from build123d import *

# Parameters (mm, degrees)
F0_W          = 10
F0_H          = 18
F1_DEPTH      = 25
F2_R          = 3.2
F3_DEPTH      = 50.401
F3_DEPTH_BACK = 35.001
F2_R_2        = 5.2
F4_DEPTH      = 5
F4_DEPTH_BACK = 35.001
F5_R          = 3.2
F6_DEPTH      = 5
F7_R          = 2
F8_SIZE       = 0.5


with BuildPart() as f1:
    # F0 (on Top) → F1 (new body)
    with BuildSketch(Plane.XY):
        Polygon((-15.2, 15.2), (15.2, 15.2), (15.2, -33.2), (25.2, -33.2), (25.2, 25.2), (-25.2, 25.2), (-25.2, -33.2), (-15.2, -33.2), align=None)
        Polygon((-15.2, -43.2), (-15.2, -33.2), (-25.2, -33.2), (-50.2, -33.2), (-60.2, -33.2), (-60.2, -43.2), align=None)
        with Locations((-55.2, -24.2)):
            Rectangle(F0_W, F0_H)
    extrude(amount=F1_DEPTH)

    # F2 (on face) → F3 (cut, two sides)
    with BuildSketch(Plane(origin=(-25.2, 0, 0), x_dir=(0, -1, 0), z_dir=(-1, 0, 0))) as f3_sk:
        with Locations((25.2, 12.5)):
            Circle(F2_R)
    extrude(amount=-F3_DEPTH, mode=Mode.SUBTRACT)
    extrude(f3_sk.sketch, amount=F3_DEPTH_BACK, mode=Mode.SUBTRACT)

    # F2 (on face) → F4 (cut, two sides)
    with BuildSketch(Plane(origin=(-25.2, 0, 0), x_dir=(0, -1, 0), z_dir=(-1, 0, 0))) as f4_sk:
        with Locations((25.2, 12.5)):
            Circle(F2_R_2)
        with Locations((25.2, 12.5)):
            Circle(F2_R, mode=Mode.SUBTRACT)
    extrude(amount=-F4_DEPTH, mode=Mode.SUBTRACT)
    extrude(f4_sk.sketch, amount=F4_DEPTH_BACK, mode=Mode.SUBTRACT)

    # F5 (on face) → F6 (cut)
    with BuildSketch(Plane.YZ.offset(25.2)):
        Polygon((-30.3, 9.5555136271), (-25.2, 6.6110272543), (-20.1, 9.5555136271), (-20.1, 15.4444863729), (-25.2, 18.3889727457), (-30.3, 15.4444863729), align=None)
        with Locations((-25.2, 12.5)):
            Circle(F5_R, mode=Mode.SUBTRACT)
    extrude(amount=-F6_DEPTH, mode=Mode.SUBTRACT)

    # F7
    f7_edges = [f1.edges().sort_by_distance(p)[0] for p in [
        (-25.2, -33.2, 12.5),
        (-15.2, -43.2, 12.5),
        (15.2, -33.2, 12.5),
        (25.2, -33.2, 12.5),
        (25.2, 25.2, 12.5),
        (-50.2, -33.2, 12.5),
        (-50.2, -15.2, 12.5),
        (-60.2, -15.2, 12.5),
        (-60.2, -43.2, 12.5),
        (-25.2, 25.2, 12.5),
    ]]
    fillet(f7_edges, radius=F7_R)

    # F8
    f8_edges = [f1.edges().sort_by_distance(p)[0] for p in [
        (15.2, -8, 25),
        (15.785786, -32.614214, 25),
        (0, 15.2, 25),
        (20.2, -33.2, 25),
        (-15.2, -13, 25),
        (24.614214, -32.614214, 25),
        (-15.785786, -42.614214, 25),
        (25.2, -4, 25),
        (-37.7, -43.2, 25),
        (24.614214, 24.614214, 25),
        (-59.614214, -42.614214, 25),
        (0, 25.2, 25),
        (-60.2, -29.2, 25),
        (-24.614214, 24.614214, 25),
        (-59.614214, -15.785786, 25),
        (-25.2, -4, 25),
        (-55.2, -15.2, 25),
        (-25.785786, -32.614214, 25),
        (-50.785786, -15.785786, 25),
        (-37.7, -33.2, 25),
        (-50.2, -24.2, 25),
        (-49.614214, -32.614214, 25),
        (15.2, -8, 0),
        (15.785786, -32.614214, 0),
        (0, 15.2, 0),
        (20.2, -33.2, 0),
        (-15.2, -13, 0),
        (24.614214, -32.614214, 0),
        (-15.785786, -42.614214, 0),
        (25.2, -4, 0),
        (-37.7, -43.2, 0),
        (24.614214, 24.614214, 0),
        (-59.614214, -42.614214, 0),
        (0, 25.2, 0),
        (-60.2, -29.2, 0),
        (-24.614214, 24.614214, 0),
        (-59.614214, -15.785786, 0),
        (-25.2, -4, 0),
        (-55.2, -15.2, 0),
        (-25.785786, -32.614214, 0),
        (-50.785786, -15.785786, 0),
        (-37.7, -33.2, 0),
        (-50.2, -24.2, 0),
        (-49.614214, -32.614214, 0),
    ]]
    chamfer(f8_edges, length=F8_SIZE)


solid = f1.part
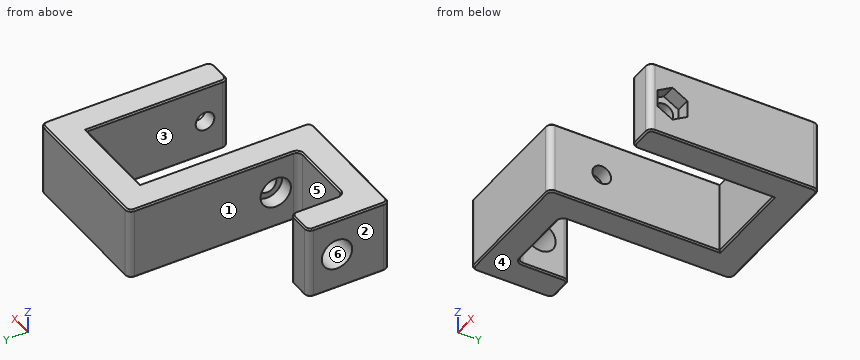
Geometry: final body of the model. Coordinates: model frame, mm. Face numbers are marked on the shaded views. A direction names the side the tool comes from. Give positions to 0.01 mm unless a question says otherwise; leave off trailing zeros. Loops run counter-clockwise (first coordinate to the right, second up) from the corner with the lowest first, then second, coordinate; pieces in that order, holes last. Notation, with made-up numbers: (-32.75, 82) - (-2.75, 82) arc R17 ccw to (-2.75, 105) - close; hole circle Ø8 at (63.5, 68.25). An arc over 180 degrees is marked (long way). One line per question, with ' | ' between items. Start each with the question number.
(1) Ray query, line 1 (X direction, y = -19.5, z = 21); line 2 (Y direction, x = 19, z = 12.5); line 3 (Y direction, x = -55.5, z = 12.5). Return the intervals inside material, ascending. Write a range as from..to.
(2) Section query A-A on y = -9.5. Return loops of the section in (x, z).
(3) Contact query for flat-ended pins moving along their axis: pin 1 (3 mm diameter, centred on y = -26.5, z = 11, fed in from -X); pin 2 (1 mm diameter, centred on y = 0, z = 12.5, fed in from -X); pin 3 (1.8 mm diameter, centred on x = 19.5, z = 7, fed in from -Y); pin 4 (6 mm diameter, centred on x = -31, y = -2.5, fed in from -Z). Output: stop coordinate, or through.
(4) Section query B-B on z = 12.5. Count the separate pieces of the cut face and the enclosed holes in it, then the cut area to 3 significant figures.
(5) Section query C-C on x = -39. Return loops of the section in (y, z), then the cut area to 4 significant figures.
(6) Section query D-D on y = 19. Return loops of the section in (x, z), then the cut area to 3 significant figures.
(7) Pull-direction query (Z, two-part tool) for the marked faces 4, 5 and 6; classes: released by +Z, released by -Z, zero draft, split by the parting line, or undercut.
(8) Reachability of the marked faces 1, 2 and 3 from +Z, -Z, +X, -X, +Y, -Y: full face, straight path, thin tool, end or side. Return the list, or none.
The answers:
1) line 1: -60.2..-50.2, -25.2..-15.2, 15.2..25.2 | line 2: -33.2..-28.4, -22..25.2 | line 3: -43.2..-30.4, -20..-15.2
2) outline: (-25.2, 0.5) - (-24.7, 0) - (-15.7, 0) - (-15.2, 0.5) - (-15.2, 24.5) - (-15.7, 25) - (-24.7, 25) - (-25.2, 24.5) - close; (15.2, 0.5) - (15.7, 0) - (24.7, 0) - (25.2, 0.5) - (25.2, 24.5) - (24.7, 25) - (15.7, 25) - (15.2, 24.5) - close
3) pin 1: x = -20.2 | pin 2: x = -25.2 | pin 3: y = -33.2 | pin 4: through
4) separate pieces: 4 | enclosed holes: 0 | area: 1,830 mm2
5) outline: (-43.2, 0.5) - (-42.7, 0) - (-33.7, 0) - (-33.2, 0.5) - (-33.2, 24.5) - (-33.7, 25) - (-42.7, 25) - (-43.2, 24.5) - close | area: 249.5 mm2
6) outline: (-25.2, 0.5) - (-24.7, 0) - (24.7, 0) - (25.2, 0.5) - (25.2, 24.5) - (24.7, 25) - (-24.7, 25) - (-25.2, 24.5) - close | area: 1,260 mm2
7) face 4: released by -Z | face 5: zero draft | face 6: undercut
8) face 1: +Z, -Z, +Y | face 2: +Z, -Z, -X, +Y, -Y | face 3: +Z, -Z, -Y
